from build123d import *

# Parameters (mm, degrees)
BOSS_EXTRUDE3_START = 40
BOSS_EXTRUDE3_DEPTH = 4
SKETCH3_W           = 5.009740145
SKETCH3_H           = 44.698182912
BOSS_EXTRUDE4_DEPTH = 2
BOSS_EXTRUDE5_DEPTH = 5
SKETCH7_W           = 62.374089496
SKETCH7_H           = 4.444300198
BOSS_EXTRUDE6_DEPTH = 10
SKETCH8_R           = 3.68
CUT_EXTRUDE1_DEPTH  = 10
BOSS_EXTRUDE7_DEPTH = 2
FILLET1_R           = 5


with BuildPart() as part:
    # Sketch4 → Boss-Extrude3 (new body)
    with BuildSketch(Plane.XY.offset(BOSS_EXTRUDE3_START)):
        Polygon((82.266178214, 7.62), (82.696382378, 7.62), (83.657798078, 0), (83.657798078, -1.756584044), (77.202578377, -1.756584044), (77.256438069, 0), (82.266178214, 0), align=None)
    extrude(amount=BOSS_EXTRUDE3_DEPTH)

    # Sketch3 → Boss-Extrude4 (add)
    with BuildSketch(Plane(origin=(0, 0, 0), x_dir=(1, 0, 0), z_dir=(0, 1, 0))):
        with Locations((79.761308141, -22.142555967)):
            Rectangle(SKETCH3_W, SKETCH3_H)
    extrude(amount=-BOSS_EXTRUDE4_DEPTH)

    # Sketch6 → Boss-Extrude5 (add)
    with BuildSketch(Plane.XY.offset(44.491647423)):
        Polygon((77.256438069, -2), (77.256438069, -3.040359502), (77.256438069, -62.213081923), (67.137259184, -75.509161123), (66.697097711, -75.509161123), (66.697097711, -80.05237461), (92.826264311, -80.05237461), (92.826264311, -75.509161123), (92.244616978, -75.509161123), (82.266178214, -2), align=None)
    extrude(amount=-BOSS_EXTRUDE5_DEPTH)

    # Sketch7 → Boss-Extrude6 (add)
    with BuildSketch(Plane.XY.offset(44.491647423)):
        with Locations((79.043692129, -77.830224511)):
            Rectangle(SKETCH7_W, SKETCH7_H)
    extrude(amount=-BOSS_EXTRUDE6_DEPTH)

    # Sketch8 → Cut-Extrude1 (cut)
    with BuildSketch(Plane(origin=(0, -75.608074412, 0), x_dir=(1, 0, 0), z_dir=(0, 1, 0))):
        with Locations(Location((53.253735199, -39.491647423, 0), (0, 0, 270))):
            Circle(SKETCH8_R)
        with Locations(Location((104.053735199, -39.491647423, 0), (0, 0, 270))):
            Circle(SKETCH8_R)
    extrude(amount=-CUT_EXTRUDE1_DEPTH, mode=Mode.SUBTRACT)

    # Sketch9 → Boss-Extrude7 (add)
    with BuildSketch(Plane(origin=(82.266178214, 0, 0), x_dir=(0, 0, -1), z_dir=(1, 0, 0))):
        Polygon((-24.429530022, -2), (-33.920992071, -14.725861543), (-39.491647423, -56.549410739), (-39.491647423, -2), align=None)
    extrude(amount=-BOSS_EXTRUDE7_DEPTH)

    # Fillet1
    # the kernel refuses this fillet: 5 mm, written as the material it adds along each edge
    with BuildSketch(Plane(origin=(82.266178214, -69.049410739, 39.491647423), x_dir=(0, 0, -1), z_dir=(0, 1, 0))) as fillet1_piece_1_section:
        with BuildLine():
            CenterArc((FILLET1_R, -FILLET1_R), FILLET1_R, 90, 90)
            Line((0, -FILLET1_R), (0, 0))
            Line((0, 0), (FILLET1_R, 0))
        make_face()
    fillet1_piece_1 = extrude(amount=79.549410739, mode=Mode.PRIVATE)
    fillet1_piece_1 = split(fillet1_piece_1, bisect_by=Plane(origin=(91.203068258, -67.836280176, 39.491647423), z_dir=(-0.9909121640469413, -0.13451053172078273, 0)), keep=Keep.TOP, mode=Mode.PRIVATE)
    fillet1_piece_1 = split(fillet1_piece_1, bisect_by=Plane(origin=(82.266178214, -68.831517537, 41.127553158), z_dir=(0, 0.13202823988691362, 0.9912459552867612)), keep=Keep.TOP, mode=Mode.PRIVATE)
    add(fillet1_piece_1)
    with BuildSketch(Plane(origin=(82.266178214, -2, 24.429530022), x_dir=(0, 0, -1), z_dir=(-1, 0, 0))) as fillet1_piece_2:
        with BuildLine():
            CenterArc((FILLET1_R * 0.501668266059, FILLET1_R), FILLET1_R, 216.717064356, 53.282935644)
            Line((-FILLET1_R * 0.299929352407, FILLET1_R * 0.402136087333), (0, 0))
            Line((0, 0), (FILLET1_R * 0.501668266059, 0))
        make_face()
    extrude(amount=2)
    with BuildSketch(Plane(origin=(82.266178214, -14.725861543, 33.920992071), x_dir=(0, 0.8015976184662758, -0.5978639126667499), z_dir=(-1, 0, 0))) as fillet1_piece_3:
        with BuildLine():
            CenterArc((FILLET1_R * 0.259830628617, FILLET1_R), FILLET1_R, 240.869747944, 29.130252056)
            Line((-FILLET1_R * 0.226966033962, FILLET1_R * 0.126484682847), (0, 0))
            Line((0, 0), (FILLET1_R * 0.259830628617, 0))
        make_face()
    extrude(amount=2)
    with BuildSketch(Plane(origin=(80.266178214, -68.016446568, 39.491647423), x_dir=(-1, 0, 0), z_dir=(0, 1, 0))) as fillet1_piece_4_section:
        with BuildLine():
            CenterArc((5, -4.586814331), FILLET1_R, 113.456454131, 66.543545869)
            Line((0, -4.586814331), (0, 0))
            Line((0, 0), (3.009740145, 0))
        make_face()
    fillet1_piece_4 = extrude(amount=66.016446568, mode=Mode.PRIVATE)
    fillet1_piece_4 = split(fillet1_piece_4, bisect_by=Plane(origin=(80.266178214, -67.816559436, 40.992366597), z_dir=(0, 0.13202823988691362, 0.9912459552867612)), keep=Keep.TOP, mode=Mode.PRIVATE)
    add(fillet1_piece_4)
    with BuildSketch(Plane(origin=(77.256438069, -62.213081923, 44.491647423), x_dir=(0, 1, 0), z_dir=(0, 0, -1))) as fillet1_piece_5:
        with BuildLine():
            CenterArc((FILLET1_R * 0.337251278502, -FILLET1_R), FILLET1_R, 90, 37.273488701)
            Line((-FILLET1_R * 0.268368983809, -FILLET1_R * 0.204246207751), (0, 0))
            Line((0, 0), (FILLET1_R * 0.337251278502, 0))
        make_face()
    extrude(amount=5)
    with BuildSketch(Plane(origin=(66.697097711, -75.608074412, 39.491647423), x_dir=(0, 1, 0), z_dir=(1, 0, 0))) as fillet1_piece_6_section:
        with BuildLine():
            CenterArc((FILLET1_R, -FILLET1_R), FILLET1_R, 90, 90)
            Line((0, -FILLET1_R), (0, 0))
            Line((0, 0), (FILLET1_R, 0))
        make_face()
    fillet1_piece_6 = extrude(amount=26.1291666, mode=Mode.PRIVATE)
    fillet1_piece_6 = split(fillet1_piece_6, bisect_by=Plane(origin=(66.697097711, -75.509161123, 39.491647423), z_dir=(0, -1, 0)), keep=Keep.TOP, mode=Mode.PRIVATE)
    add(fillet1_piece_6)
    with BuildSketch(Plane(origin=(54.197097711, -75.608074412, 39.491647423), x_dir=(0, 1, 0), z_dir=(1, 0, 0))) as fillet1_piece_7_section:
        with BuildLine():
            CenterArc((FILLET1_R, -FILLET1_R), FILLET1_R, 90, 90)
            Line((0, -FILLET1_R), (0, 0))
            Line((0, 0), (FILLET1_R, 0))
        make_face()
    fillet1_piece_7 = extrude(amount=51.1291666, mode=Mode.PRIVATE)
    fillet1_piece_7 = split(fillet1_piece_7, bisect_by=Plane(origin=(91.569404015, -70.535002372, 39.491647423), z_dir=(-0.9909121640469413, -0.13451053172078273, 0)), keep=Keep.TOP, mode=Mode.PRIVATE)
    fillet1_piece_7 = split(fillet1_piece_7, bisect_by=Plane(origin=(62.343451037, -81.807977807, 39.491647423), z_dir=(0.7957537922487953, -0.6056202623110138, 0)), keep=Keep.TOP, mode=Mode.PRIVATE)
    add(fillet1_piece_7)
    # the kernel refuses this fillet: 5 mm, written as the material it takes off along each edge
    with BuildSketch(Plane(origin=(47.856647381, -92.55237461, 34.491647423), x_dir=(1, 0, 0), z_dir=(0, 1, 0))) as fillet1_2_piece_1:
        with BuildLine():
            CenterArc((FILLET1_R, -FILLET1_R), FILLET1_R, 90, 90)
            Line((0, -FILLET1_R), (0, 0))
            Line((0, 0), (FILLET1_R, 0))
        make_face()
    extrude(amount=29.444300198, mode=Mode.SUBTRACT)
    with BuildSketch(Plane(origin=(110.230736877, -63.108074412, 34.491647423), x_dir=(0, 0, 1), z_dir=(0, -1, 0))) as fillet1_2_piece_2:
        with BuildLine():
            CenterArc((FILLET1_R, FILLET1_R), FILLET1_R, 180, 90)
            Line((0, FILLET1_R), (0, 0))
            Line((0, 0), (FILLET1_R, 0))
        make_face()
    extrude(amount=29.444300198, mode=Mode.SUBTRACT)


solid = part.part
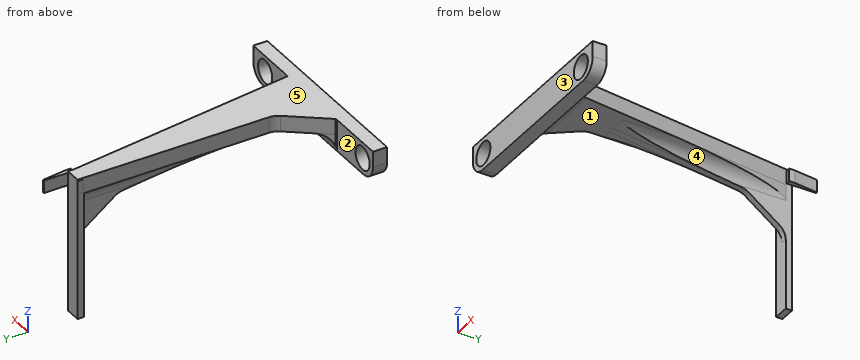
CAD build for the part. Positions are in the model's coordinates, mm. Face numbers are marked on the shaded views. A direction names the side the tool comes from. Give positions to 0.01 mm unless a question says otherwise; leave off trailing zeros. Write each loop counter-clockwise with the first axis right and the second up, starting at its lowest first coordinate (ties: lowest second). Pieces come first, ordered by that corner, then holes. Notation, with made-up numbers: M -40,0 L 10,0 A10 ccw 10,16 Z; hole C -9.5,60 d9. An arc over 180 degrees is marked long. Put each result on its own line as item: value. Start each with the question number.
(1) Mould opens along Y. For the marked faces 1, 2 and 3 say: +Y half, -Y half, draft (parallel to the pull), parting line (faces both ways), or undercut.
(2) Band-saw the part on C-C, the plane z = 31.5. Write the cut outline in (x, y), and give its area (3 significant figures).
(3) Band-saw the part on B-B, the plane y = -5.5. Write the cut outline in (x, z).
(4) Flat gauge pins, fed straight in: pin 1 Ø14.5 at (y, z) = (-14.5, 31) entering from -X; pin 2 Ø12 at (x, z) = (68.5, 17.5) entering from -Y; pin 3 Ø1.5 at (x, y) = (82.5, 3) entering from -Z; pin 4 Ø12 at (x, y) = (72, -47.5) entering from -Z. Where does each tip first touch, or does it go through?
(5) Band-saw the part on A-A, the plane x = 102. Write the cut outline in (y, z), and give its area (3 significant figures).
(6) Which spindle directions (+Z, -Z, +X, -X, +Y, -Y) get a long thin tool onto all of the face, cutting with end or side? Do the marked faces 4 and 5. Say none if no direction does.
(7) Probe L1, parallel to Y at x = 80, z = 25.5; L2, parallel to Y at x = 60.5, z = 35; L3, parallel to X at y = -71.5, z = 40. List the from-to ranges inside material, lowest first.
(8) Band-saw the part on D-D, the plane x = 89. Write the cut outline in (y, z), and give its area (3 significant figures).
Response values:
1. face 1: undercut
1. face 2: +Y half
1. face 3: -Y half
2. outline: M 77.26,-2 L 80.27,-2 L 80.27,-11.48 L 82.27,-11.48 L 82.27,0 L 77.26,0 Z
2. area: 29.0 mm2
3. outline: M 77.26,39.49 A5 cw 80.27,34.9 L 80.27,27.04 L 82.27,27.04 L 82.27,34.49 A5 cw 82.74,36.62 L 82.74,44.49 L 77.26,44.49 Z
4. pin 1: stops at x = 78.98
4. pin 2: passes through
4. pin 3: stops at z = 40
4. pin 4: stops at z = 39.09
5. outline: M -80.05,34.49 L -75.61,34.49 L -75.61,36.44 L -80.05,36.44 Z; M -80.05,42.55 L -75.61,42.55 L -75.61,44.49 L -80.05,44.49 Z
5. area: 17.3 mm2
6. face 4: -Z, +X, +Y
6. face 5: +Z, +X, -X, +Y, -Y
7. L1: y = -2 to 0
7. L2: y = -80.05 to -75.61
7. L3: x = 70.19 to 91.7
8. outline: M -80.05,34.49 L -75.61,34.49 A5 cw -70.61,39.49 L -51.61,39.49 L -51.61,44.49 L -80.05,44.49 Z
8. area: 170 mm2
